Source: CAD feature listing. Evaluate the final solid. Frame: model axes, mm. Face numbers are marked on the shaded views. A direction names the side the tool comes from. Coordinates: 2 decimals unless noted, no trailing zeros. Write each loop counter-clockwise with the first axis right and the second up, starting at its lowest first coordinate (ties: lowest second). Pieces come first, ordered by that corner, then holes. Notation, with made-up numbers: (18, -37) -> (51, -37) arc R20 ccw to (51, -30) -> close; hole circle Ø7 at (32, -25). An arc over 180 degrees is marked (long way). One line per item, written item: value. Start each with the question number.
1. Section query D-D, the plane z = -6.35. Output: boundary loops of the cut face in (x, y) (3 decimals).
2. Access query for the marked faces 4 and 5. Directions: +Z, -Z, +X, -X, +Y, -Y. A direction counts if a zero-diameter tool reaches every point of the face in a straight line with its end or side. Return the directions, or none.
3. Section query B-B, the plane z = -2. Output: boundary loops of the cut face in (x, y) (3 decimals).
4. Mould query, pull axis Z, two halves, no side actions, for the marked faces 1, 2 and 3. Classes: released by +Z, released by -Z, zero draft, split by the parting line, or undercut.
5. Section query A-A, the plane y = 0.4. Output: boundary loops of the cut face in (x, z) (3 decimals), and give its area (3 significant figures).
6. First-contact query: P1, Ø1, axis at x = 3.5, z = -8.5, coming from the +Y side. Flat tip, straight axial feed; report the tip coordinate or a pass-through.
7. Line query: line 1 (Z direction, x = 6.5, y = 0.2) (3 decimals); line 2 (X direction, y = 1.8, z = -5) (3 decimals); line 3 (Z direction, x = 7.5, y = 1) (3 decimals). Output: solid intervals per line, ascending.
8. Section query C-C, the plane x = 2.5. Output: boundary loops of the cut face in (y, z) (3 decimals), and give its area (3 significant figures).
from build123d import *

# Parameters (mm, degrees)
SKETCH1_W           = 12.7
SKETCH1_H           = 12.7
BOSS_EXTRUDE1_DEPTH = 2.54
FILLET1_R           = 0.635
SHELL1_START        = 0.635
SHELL1_OUTLINE_W    = 1.905
SHELL1_OUTLINE_H    = 11.43
SHELL1_DEPTH        = 11.43
SKETCH2_R           = 2.54
BOSS_EXTRUDE2_DEPTH = 1.905
BOSS_EXTRUDE4_DEPTH = 0.00254


# Read off the part's stored shape, not the designer's step: Shell1
with BuildPart() as part:
    # Sketch1 → Boss-Extrude1 (new body)
    with BuildSketch(Plane(origin=(0, 0, 0), x_dir=(1, 0, 0), z_dir=(0, 1, 0))):
        with Locations((6.35, 6.35)):
            Rectangle(SKETCH1_W, SKETCH1_H)
    extrude(amount=BOSS_EXTRUDE1_DEPTH)

    # Fillet1
    fillet1_edges = [part.edges().sort_by_distance(p)[0] for p in [
        (0, 1.27, -12.7),
        (12.7, 1.27, -12.7),
        (12.7, 1.27, 0),
        (0, 1.27, 0),
    ]]
    fillet(fillet1_edges, radius=FILLET1_R)

    # Shell1 outline → Shell1 (cut)
    with BuildSketch(Plane.YZ.offset(SHELL1_START)):
        with Locations((0.9525, -6.35)):
            Rectangle(SHELL1_OUTLINE_W, SHELL1_OUTLINE_H)
    extrude(amount=SHELL1_DEPTH, mode=Mode.SUBTRACT)

    # Sketch2 → Boss-Extrude2 (add)
    with BuildSketch(Plane(origin=(0, 1.905, 0), x_dir=(-1, 0, 0), z_dir=(0, -1, 0))):
        with Locations(Location((-6.35, 6.35, 0), (0, 0, 270))):
            Circle(SKETCH2_R)
    extrude(amount=BOSS_EXTRUDE2_DEPTH)

    # Sketch4 → Boss-Extrude4 (add)
    # profile 1 of 2: a face of its own
    with BuildSketch(Plane(origin=(0, 2.54, 0), x_dir=(1, 0, 0), z_dir=(0, 1, 0))):
        with BuildLine():
            Line((6.359463942, 2.585589744), (5.854465946, 2.839996795))
            Line((5.854465946, 2.839996795), (6.407801282, 3.928858974))
            add(Edge.make_bspline(
                [(6.407801282, 3.928858974), (6.37510896, 3.929692258), (6.310926022, 3.931328196), (6.216421654, 3.944922824), (6.126049401, 3.968129722), (6.038744074, 3.999023949), (5.955713077, 4.040440861), (5.875949592, 4.089869773), (5.800557817, 4.1492579), (5.72918427, 4.21601261), (5.664017941, 4.289798172), (5.607454945, 4.369153296), (5.558153789, 4.452064974), (5.519814505, 4.540404997), (5.489020198, 4.632526927), (5.466520324, 4.728907598), (5.45389399, 4.829969864), (5.452129186, 4.898751737), (5.451230769, 4.933766827)],
                knots=[0, 0, 0, 0, 1.014336294, 1.991387562, 2.955278539, 3.906441712, 4.859855302, 5.829322156, 6.813833455, 7.833278715, 8.858926674, 9.863225732, 10.85404919, 11.846815163, 12.845559416, 13.865450493, 14.913355531, 16, 16, 16, 16], degree=3))
            add(Edge.make_bspline(
                [(5.451230769, 4.933766827), (5.4520641, 4.967731119), (5.45370616, 5.034657053), (5.467343628, 5.132882545), (5.48978737, 5.227193368), (5.520579382, 5.317573499), (5.561571384, 5.40341349), (5.60955148, 5.486057396), (5.66820497, 5.563795404), (5.734463459, 5.636964041), (5.80697986, 5.703900425), (5.883913674, 5.762753864), (5.964915094, 5.811949684), (6.048943173, 5.853265097), (6.137516777, 5.884133404), (6.229355921, 5.907423313), (6.325144744, 5.920864918), (6.3901642, 5.922555021), (6.423065705, 5.923410256)],
                knots=[0, 0, 0, 0, 1.055538678, 2.079917126, 3.075849687, 4.065898488, 5.041806164, 6.028602842, 7.031727914, 8.062953097, 9.093756959, 10.095582084, 11.068815425, 12.035667573, 13.000833448, 13.979119574, 14.977382875, 16, 16, 16, 16], degree=3))
            add(Edge.make_bspline(
                [(6.423065705, 5.923410256), (6.457468209, 5.922702118), (6.525116079, 5.92130966), (6.624143475, 5.905944432), (6.71888888, 5.882371363), (6.809737259, 5.850354325), (6.895560767, 5.806900578), (6.977077532, 5.754820959), (7.054016404, 5.692963174), (7.125551114, 5.623110154), (7.190611134, 5.547131925), (7.248278747, 5.467601049), (7.296721989, 5.384673031), (7.336399968, 5.299087975), (7.367308914, 5.210711801), (7.388554875, 5.119419152), (7.402659837, 5.025366142), (7.4042647, 4.961591251), (7.405076923, 4.929314704)],
                knots=[0, 0, 0, 0, 1.062826075, 2.08990367, 3.089830715, 4.078784409, 5.060762809, 6.057138927, 7.064407536, 8.107320944, 9.143871033, 10.153461498, 11.140480137, 12.108246174, 13.065926856, 14.029354859, 15.002654194, 16, 16, 16, 16], degree=3))
            add(Edge.make_bspline(
                [(7.405076923, 4.929314704), (7.404633685, 4.904698148), (7.403740905, 4.855114869), (7.39496241, 4.780759368), (7.381643664, 4.706197784), (7.36618444, 4.643509984), (7.349977595, 4.590667976), (7.334206488, 4.545841333), (7.313971695, 4.496075342), (7.291377525, 4.441036433), (7.265210817, 4.38096596), (7.234929053, 4.316151081), (7.202362379, 4.245630527), (7.178357526, 4.197409534), (7.165934295, 4.172453726)],
                knots=[0, 0, 0, 0, 1.105131805, 2.225983929, 3.357782449, 4.505488967, 5.122909461, 5.839607681, 6.638776516, 7.535249922, 8.51168636, 9.581005249, 10.748097757, 12, 12, 12, 12], degree=3))
            Line((7.165934295, 4.172453726), (6.359463942, 2.585589744))
        make_face()
        with BuildLine():
            add(Edge.make_bspline(
                [(6.435786058, 4.458025641), (6.46309194, 4.459633217), (6.516441451, 4.462774058), (6.593074476, 4.487059704), (6.661657137, 4.528619041), (6.722444439, 4.583831174), (6.772677205, 4.651192501), (6.809199713, 4.727877384), (6.831696453, 4.812297764), (6.834013104, 4.871082471), (6.835205128, 4.901329928)],
                knots=[0, 0, 0, 0, 0.984774978, 1.924027336, 2.867853169, 3.859505234, 4.871392407, 5.881338128, 6.909850265, 8, 8, 8, 8], degree=3))
            add(Edge.make_bspline(
                [(6.835205128, 4.901329928), (6.833769465, 4.932206601), (6.830976757, 4.992269104), (6.808264507, 5.078715896), (6.76945384, 5.156858669), (6.716654147, 5.224786259), (6.655011194, 5.281632973), (6.586078813, 5.323157968), (6.511530825, 5.348835693), (6.45994101, 5.351960048), (6.433878005, 5.353538462)],
                knots=[0, 0, 0, 0, 1.104110315, 2.147758178, 3.172670271, 4.206310416, 5.210906102, 6.157051016, 7.068948237, 8, 8, 8, 8], degree=3))
            add(Edge.make_bspline(
                [(6.433878005, 5.353538462), (6.406330871, 5.351999712), (6.3522423, 5.348978389), (6.274657461, 5.323362327), (6.203136419, 5.282634751), (6.140678718, 5.225595158), (6.086623972, 5.158562153), (6.048930123, 5.080155613), (6.025083687, 4.99431208), (6.022453466, 4.934141867), (6.021102564, 4.903237981)],
                knots=[0, 0, 0, 0, 0.970967322, 1.90648639, 2.855811969, 3.858352357, 4.877096915, 5.878517833, 6.91039038, 8, 8, 8, 8], degree=3))
            add(Edge.make_bspline(
                [(6.021102564, 4.903237981), (6.022513665, 4.872774607), (6.025258108, 4.813526525), (6.048259331, 4.728627364), (6.085726018, 4.651536658), (6.136945653, 4.583644091), (6.20003563, 4.528159923), (6.271669441, 4.487043277), (6.3515753, 4.462708207), (6.407210509, 4.459614594), (6.435786058, 4.458025641)],
                knots=[0, 0, 0, 0, 1.075706617, 2.092137047, 3.084482865, 4.090466434, 5.0784141, 6.035155512, 6.990809768, 8, 8, 8, 8], degree=3))
        make_face(mode=Mode.SUBTRACT)
    # profile 2 of 2: a face of its own
    with BuildSketch(Plane(origin=(0, 2.54, 0), x_dir=(1, 0, 0), z_dir=(0, 1, 0))):
        with BuildLine():
            Line((6.128386018, 11.257410256), (6.840089744, 11.257410256))
            add(Edge.make_bspline(
                [(6.840089744, 11.257410256), (6.809822419, 11.222311467), (6.749724305, 11.152620105), (6.666795677, 11.043407385), (6.58880222, 10.932667564), (6.516859259, 10.819319518), (6.450831014, 10.703557736), (6.390172367, 10.585956901), (6.336053768, 10.465927477), (6.287531103, 10.343512884), (6.244695572, 10.21769031), (6.207842411, 10.087755624), (6.176795055, 9.953583531), (6.151264275, 9.815013647), (6.131654114, 9.672170871), (6.117982965, 9.524677216), (6.108469866, 9.373014933), (6.107757668, 9.270294234), (6.107397436, 9.21833774)],
                knots=[0, 0, 0, 0, 1.00236213, 1.990267575, 2.964862165, 3.931797803, 4.893137898, 5.846900052, 6.793123604, 7.740135921, 8.694427184, 9.667077551, 10.660503013, 11.672460941, 12.714089686, 13.778281025, 14.87624668, 16, 16, 16, 16], degree=3))
            add(Edge.make_bspline(
                [(6.107397436, 9.21833774), (6.107995993, 9.162143219), (6.109175923, 9.051367583), (6.118877551, 8.887757803), (6.134923993, 8.729310145), (6.155999738, 8.575722074), (6.184973215, 8.427707126), (6.219082012, 8.284484773), (6.260167582, 8.146690387), (6.292872796, 8.057661908), (6.309015024, 8.013720353)],
                knots=[0, 0, 0, 0, 1.097990858, 2.164457195, 3.201156713, 4.209415668, 5.192484095, 6.147015238, 7.085427113, 8, 8, 8, 8], degree=3))
            add(Edge.make_bspline(
                [(6.309015024, 8.013720353), (6.322859685, 7.979852544), (6.351131554, 7.910691856), (6.401423106, 7.807609383), (6.457716212, 7.702288141), (6.521502326, 7.595201452), (6.590089423, 7.484963434), (6.66788775, 7.373996815), (6.750785957, 7.259995238), (6.809954754, 7.184594376), (6.840089744, 7.146192308)],
                knots=[0, 0, 0, 0, 0.860028042, 1.756243877, 2.695094802, 3.667075869, 4.686284936, 5.746781471, 6.852423585, 8, 8, 8, 8], degree=3))
            Line((6.840089744, 7.146192308), (6.128386018, 7.146192308))
            add(Edge.make_bspline(
                [(6.128386018, 7.146192308), (6.101555843, 7.190097535), (6.048888171, 7.276283561), (5.97672167, 7.406860871), (5.908837677, 7.533983087), (5.84863606, 7.65988857), (5.79329841, 7.782919252), (5.746285673, 7.904803232), (5.702814586, 8.023514572), (5.667008208, 8.142113651), (5.636420071, 8.262084169), (5.609358218, 8.385886124), (5.587541556, 8.514997933), (5.568864716, 8.649218102), (5.555169811, 8.788642241), (5.545088524, 8.933073848), (5.538405493, 9.082591024), (5.537822099, 9.183985488), (5.537525641, 9.235510216)],
                knots=[0, 0, 0, 0, 1.119871376, 2.19830916, 3.246961562, 4.256259542, 5.235550337, 6.182491613, 7.09917337, 7.986748165, 8.877687696, 9.793695483, 10.744317876, 11.727190303, 12.742913882, 13.793068013, 14.878522868, 16, 16, 16, 16], degree=3))
            add(Edge.make_bspline(
                [(5.537525641, 9.235510216), (5.537767643, 9.285977066), (5.538244775, 9.385478056), (5.545734032, 9.532235898), (5.556506209, 9.67432497), (5.570575435, 9.81170086), (5.590786974, 9.944167937), (5.613890789, 10.072003043), (5.641993832, 10.195063696), (5.674588264, 10.314351115), (5.712537615, 10.431354955), (5.755186155, 10.548123871), (5.803610458, 10.665231326), (5.857886642, 10.78278746), (5.916995095, 10.901297384), (5.981837867, 11.020140735), (6.052595779, 11.139162984), (6.102930607, 11.217694947), (6.128386018, 11.257410256)],
                knots=[0, 0, 0, 0, 1.13127193, 2.230428031, 3.293392423, 4.325815098, 5.325330466, 6.296707414, 7.23754678, 8.15420938, 9.068070667, 9.994306547, 10.940496973, 11.908145907, 12.896524899, 13.908929949, 14.942500703, 16, 16, 16, 16], degree=3))
        make_face()
    extrude(amount=BOSS_EXTRUDE4_DEPTH)


solid = part.part
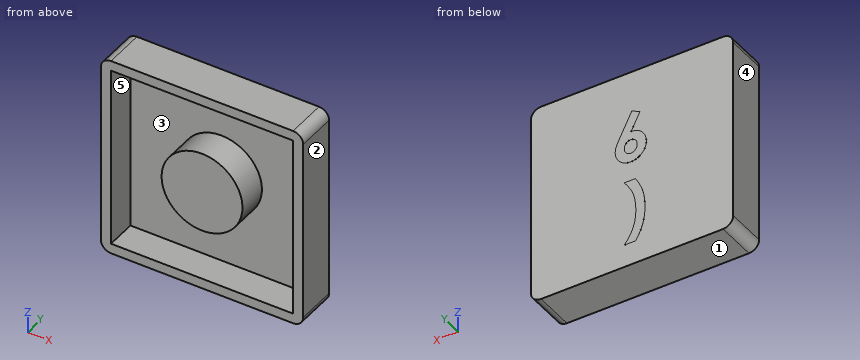
Computed values:
1. outline: (0, 0) -> (0.635, 0) -> (0.635, 1.905) -> (3.81, 1.905) -> (3.81, 0) -> (8.89, 0) -> (8.89, 1.905) -> (12.065, 1.905) -> (12.065, 0) -> (12.7, 0) -> (12.7, 2.54) -> (0, 2.54) -> close
2. face 4: +Z, -Z, -X, +Y, -Y
2. face 5: -Y
3. outline: (0, 0) -> (0.635, 0) -> (0.635, 1.905) -> (12.065, 1.905) -> (12.065, 0) -> (12.7, 0) -> (12.7, 2.54) -> (0, 2.54) -> close
4. face 1: released by -Z
4. face 2: zero draft
4. face 3: undercut
5. outline: (0, -12.065) arc R0.635 ccw to (0.635, -12.7) -> (12.065, -12.7) arc R0.635 ccw to (12.7, -12.065) -> (12.7, -0.635) arc R0.635 ccw to (12.065, 0) -> (0.635, 0) arc R0.635 ccw to (0, -0.635) -> close; circle Ø5.08 at (6.35, -6.35); hole (0.635, -12.065) -> (12.065, -12.065) -> (12.065, -0.635) -> (0.635, -0.635) -> close
5. area: 50.6 mm²
6. P1: stops at y = 2.54
7. line 1: z = -12.7 to -12.065, -8.886 to -3.814, -0.635 to 0
7. line 2: x = 0 to 0.635, 4.198 to 8.502, 12.065 to 12.7
7. line 3: z = -12.7 to -12.065, -8.615 to -4.085, -0.635 to 0
8. outline: (0, -12.7) -> (2.54, -12.7) -> (2.54, 0) -> (0, 0) -> (0, -0.635) -> (1.905, -0.635) -> (1.905, -12.065) -> (0, -12.065) -> close
8. area: 10.5 mm²
